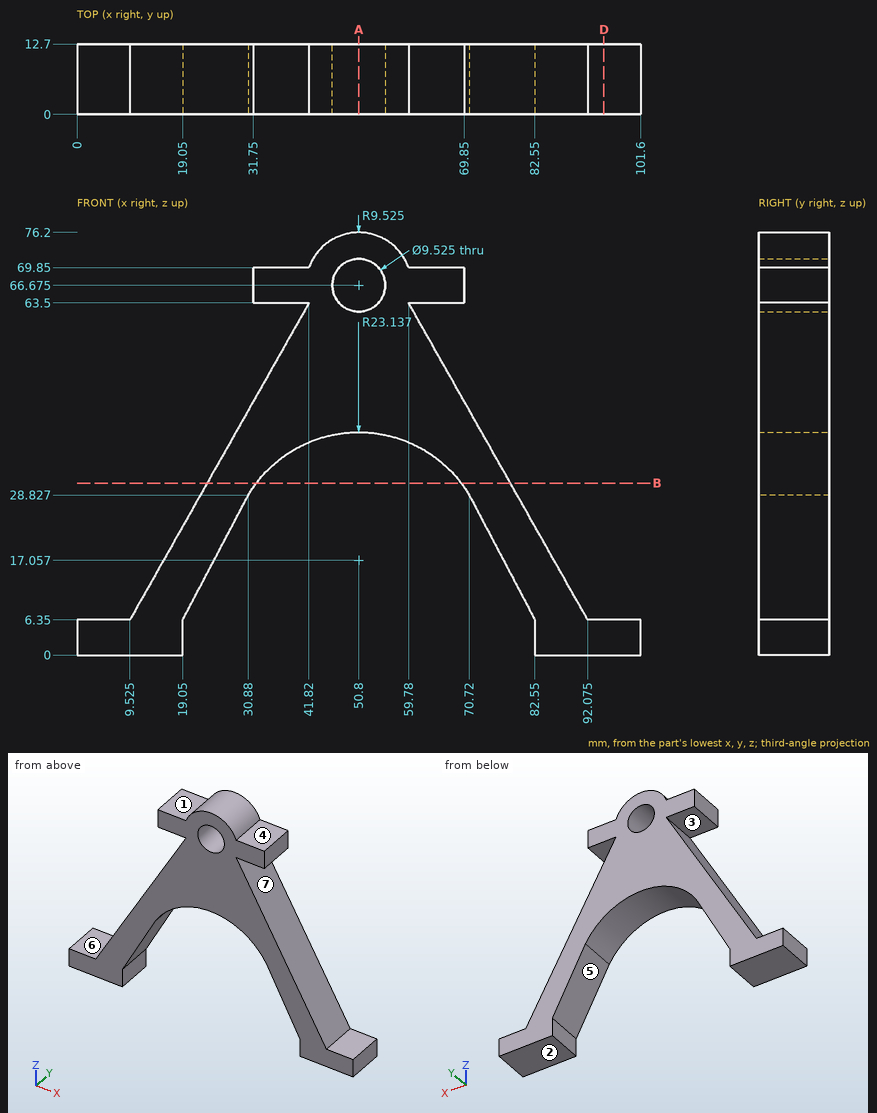
Verification items for this drawing (mm, ordinates from the low corner). A direction names the side the tool comes from. Give positions to 0.01 mm unless a question says otherwise; leave off trailing zeros. Order: outer loops, then holes, each group sorted by start corner. A loop starts at its lowest first (then second) coordinate and runs counter-clockwise, first axis right, second up.
1) Gauge pin test, flat ends, axial feed: pin 1 (7 mm diameter, centred on y = 8, z = 4.5, fed in from -X); pin 2 (5 mm diameter, centred on y = 9, z = 66.5, fed in from -X); pin 3 (2 mm diameter, centred on x = 72.5, z = 47, fed in from -Y); pin 4 (5 mm diameter, centred on y = 9, z = 67, fed in from +X). Record the tip position at first contact, or that the pin passes through.
Results are:
pin 1: stops at x = 0
pin 2: stops at x = 31.75
pin 3: passes through
pin 4: stops at x = 69.85
2) Tool access check on the marked faces 4, 5, 6 and 7. Record the directions out of +Z, -Z, +X, -X, +Y, -Y that give a thin tool (end or side, any length) a straight path to the whole face; none if there is none.
Results are:
face 4: +Z, +X, +Y, -Y
face 5: -Z, +Y, -Y
face 6: +Z, -X, +Y, -Y
face 7: +X, +Y, -Y
3) Material ranges on probe 1 along Z at (x, y) = (50.8, 5.75) (1 decimal); probe 2 along X at (y, z) = (10.25, 4); probe 3 along Z at (x, y) = (49, 11.5) (1 decimal), recorded low to high.
Results are:
probe 1: z = 40.2 to 61.9, 71.4 to 76.2
probe 2: x = 0 to 19.05, 82.55 to 101.6
probe 3: z = 40.1 to 62.3, 71.1 to 76
4) Draft check along Z on the marked faces 1, 2 and 3. Enter one of: released by +Z, released by -Z, zero draft, split by the parting line, or undercut.
Results are:
face 1: released by +Z
face 2: released by -Z
face 3: undercut
5) Cross-section at A-A (x = 50.8). Record the boundary of the cut face in (y, z) (1 decimal), then the cut area to 3 significant figures.
Results are:
outline: (0, 40.2) - (12.7, 40.2) - (12.7, 61.9) - (0, 61.9) - close; (0, 71.4) - (12.7, 71.4) - (12.7, 76.2) - (0, 76.2) - close
area: 336 mm2
6) Cross-section at B-B (z = 31). Record the boundary of the cut face in (x, y), then the cut area to 3 significant figures.
Results are:
outline: (23.45, 0) - (32.34, 0) - (32.34, 12.7) - (23.45, 12.7) - close; (69.26, 0) - (78.15, 0) - (78.15, 12.7) - (69.26, 12.7) - close
area: 226 mm2
7) Cross-section at D-D (x = 95). Record the boundary of the cut face in (y, z).
Results are:
outline: (0, 0) - (12.7, 0) - (12.7, 6.35) - (0, 6.35) - close
